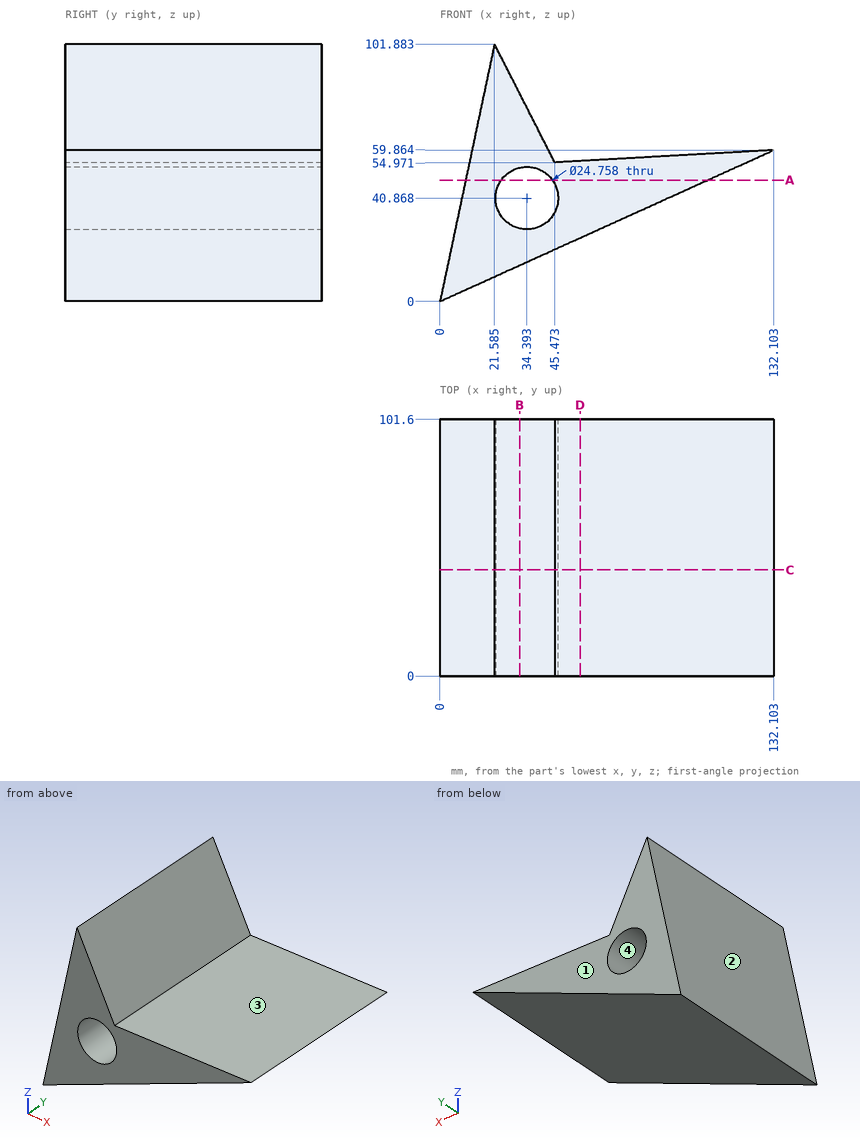
Print and shaded views of the part. All mm, measured from the part's lowest x, y and z. Coordinates: 2 decimals unless noted, no trailing zeros. Write each loop counter-clockwise with the first axis right and the second up, starting at its lowest first coordinate (ties: lowest second). Pieces come first, ordered by that corner, then holes.
(1) Two-plate mould, pull along X, no slides. Class the marked faces 1, 2, 3 and 4: +X half, -X half, draft (parallel to the pull), parting line (faces both ways), or undercut.
(2) Drill centre lines: probe 1 along Z at (x, y) = (36.5, 82.5) (1 decimal); probe 2 along X at (y, z) = (67, 34) (1 decimal); probe 3 along Z at (x, y) = (43, 22) (1 decimal). Where is each one in solid material? Low to high.
(3) Flat gauge pins, fed straight in: pin 1 (3 mm diameter, centred on y = 41, z = 15, fed in from -X); pin 2 (1 mm diameter, centred on x = 26, y = 90.5, fed in from +Z) (1 decimal); pin 3 (2 mm diameter, centred on y = 27, z = 81.5, fed in from +X). Where does each tip first touch, or does it go through?
(4) Cut at D-D, the plane x = 55.5. List the corners of the cut face in (y, z).
(5) Cut at C-C, the plane y = 42. List the corners of the cut face in (x, z) (1 decimal), and give its area (3 significant figures).
(6) Cut at A-A, the plane z = 48. List the corners of the cut face in (x, y) (1 decimal).
(7) Cut at B-B, the plane x = 31.5. List the corners of the cut face in (y, z) (1 decimal).
Geometry says:
1. face 1: draft
1. face 2: -X half
1. face 3: undercut
1. face 4: undercut
2. probe 1: z = 16.5 to 28.7, 53.1 to 72.6
2. probe 2: x = 7.2 to 24.1, 44.7 to 75
2. probe 3: z = 19.5 to 32, 49.8 to 59.8
3. pin 1: stops at x = 2.86
3. pin 2: stops at z = 94.2
3. pin 3: stops at x = 32.47
4. outline: (0, 25.15) - (101.6, 25.15) - (101.6, 55.54) - (0, 55.54) - close
5. outline: (0, 0) - (132.1, 59.9) - (45.5, 55) - (21.6, 101.9) - close; hole circle Ø24.8 at (34.4, 40.9)
5. area: 3,510 mm2
6. outline: (10.2, 0) - (24.3, 0) - (24.3, 101.6) - (10.2, 101.6) - close; (44.5, 0) - (105.9, 0) - (105.9, 101.6) - (44.5, 101.6) - close
7. outline: (0, 14.3) - (101.6, 14.3) - (101.6, 28.8) - (0, 28.8) - close; (0, 52.9) - (101.6, 52.9) - (101.6, 82.4) - (0, 82.4) - close
